Could you check a few things on this model? Use its own coordinates, in mm. A direction names the side the tool comes from. Coordinates: 2 decimals unless noted, no trailing zeros. Loops run counter-clockwise (first coordinate to the right, second up) from the corner with the lowest first, then second, coordinate; pieces in that order, holes last. Notation, with made-up numbers: (25, 67.25) - (31, 67.25) arc R5 ccw to (31, 75.25) - close; hole circle Ø6 at (68.25, 49.5). An arc over 180 degrees is marked (long way). Put each result on its own line as item: value. Start each with the question number.
```python
from build123d import *

# Parameters (mm, degrees)
SKETCH1_R           = 57
SKETCH1_R_2         = 2
SKETCH1_R_3         = 5.25
SKETCH1_R_4         = 10.75
BOSS_EXTRUDE1_DEPTH = 20
SKETCH2_R           = 57
SKETCH2_R_2         = 54
BOSS_EXTRUDE2_DEPTH = 130
SKETCH3_R           = 8
CUT_EXTRUDE1_DEPTH  = 19.5
SKETCH5_R           = 12
CUT_EXTRUDE3_DEPTH  = 6.05


with BuildPart() as part:
    # Sketch1 → Boss-Extrude1 (new body)
    with BuildSketch(Plane.XY):
        with Locations((0, 25)):
            Circle(SKETCH1_R)
        with Locations((12, 0)):
            Circle(SKETCH1_R_2, mode=Mode.SUBTRACT)
        with Locations((0, -12)):
            Circle(SKETCH1_R_2, mode=Mode.SUBTRACT)
        with Locations((-12, 0)):
            Circle(SKETCH1_R_2, mode=Mode.SUBTRACT)
        Circle(SKETCH1_R_3, mode=Mode.SUBTRACT)
        with Locations((0, 12)):
            Circle(SKETCH1_R_2, mode=Mode.SUBTRACT)
        with Locations((0, 50)):
            Circle(SKETCH1_R_4, mode=Mode.SUBTRACT)
    extrude(amount=-BOSS_EXTRUDE1_DEPTH)

    # Sketch2 → Boss-Extrude2 (add)
    with BuildSketch(Plane.XY):
        with Locations((0, 25)):
            Circle(SKETCH2_R)
        with Locations((0, 25)):
            Circle(SKETCH2_R_2, mode=Mode.SUBTRACT)
    extrude(amount=-BOSS_EXTRUDE2_DEPTH)

    # Sketch3 → Cut-Extrude1 (cut)
    with BuildSketch(Plane.XY):
        with Locations((40, 25)):
            Circle(SKETCH3_R)
    cut_extrude1 = extrude(amount=-CUT_EXTRUDE1_DEPTH, mode=Mode.SUBTRACT)

    # Sketch5 → Cut-Extrude3 (cut)
    with BuildSketch(Plane(origin=(0, 0, -20), x_dir=(-1, 0, 0), z_dir=(0, 0, -1))):
        with Locations((-40, 25)):
            Circle(SKETCH5_R)
    cut_extrude3 = extrude(amount=-CUT_EXTRUDE3_DEPTH, mode=Mode.SUBTRACT)

    # Mirror1: Cut-Extrude1, Cut-Extrude3 across plane
    add(cut_extrude1.mirror(Plane(origin=(0, 0, 0), x_dir=(0, 0, 1), z_dir=(1, 0, 0))), mode=Mode.SUBTRACT)
    add(cut_extrude3.mirror(Plane(origin=(0, 0, 0), x_dir=(0, 0, 1), z_dir=(1, 0, 0))), mode=Mode.SUBTRACT)


solid = part.part
```
(1) I want a section at A-A on x = 0. List the corners of the cut face in (y, z) for me.
(2) Which directions (+Z, -Z, +X, -X, +Y, -Y) give clear straight access to the entire face, cutting with the end or side of a thin tool? Please do faces 1 (the cylindrical face through (-49.523, 17.698, -17.017)), 2 (the cylindrical face through (0, 14, -10)).
(3) I need wall thicknesses on L1, parallel to Y at x = 0, z = -10.25; L2, parallel to X at y = -1, z = -14; L3, parallel to Y at x = -1, z = -10. Which ranges of each line are inside material? Lowest first, please. Write a range as [from, to].
(4) For pin 1 Ø8 at (y, z) = (59, -96) entering from -X; pin 2 Ø9.5 at (x, y) = (-40, 25) entering from +Z; pin 3 Ø4 at (x, z) = (-24, -33) entering from +Y; pin 4 Ø6.5 at (x, y) = (-12, 0) entering from -Z, each with a flat end and sliding along its axis, tell me the tip position at first contact or that it passes through.
(5) I want a section at C-C on x = -41.5. List the corners of the cut face in (y, z) for me, and give its area (3 significant figures).
(6) I want a section at B-B on y = 41. List the corners of the cut face in (x, z) for me.
(7) I want a section at D-D on z = -92. List the corners of the cut face in (x, y) for me.
(8) If we mould it in two halves opening along X, with no side actions, what happens to faces 3 (the flat face through (32, 23, -13.95)), 4 (the cylindrical face through (-12.356, -30.645, -64.09)), 5 (the flat face through (50, 4, -130))? For each: pulls with the +X half, pulls with the -X half, needs draft (parallel to the pull), parting line crosses it, or undercut.
Answer sheet:
1. outline: (-32, -130) - (-29, -130) - (-29, -20) - (-14, -20) - (-14, 0) - (-32, 0) - close; (-10, -20) - (-5.25, -20) - (-5.25, 0) - (-10, 0) - close; (5.25, -20) - (10, -20) - (10, 0) - (5.25, 0) - close; (14, -20) - (39.25, -20) - (39.25, 0) - (14, 0) - close; (60.75, -20) - (79, -20) - (79, -130) - (82, -130) - (82, 0) - (60.75, 0) - close
2. face 1: -Z
2. face 2: +Z, -Z
3. L1: y = [-32, -14], [-10, -5.25], [5.25, 10], [14, 39.25], [60.75, 82]
3. L2: x = [-50.72, -13.73], [-10.27, -5.15], [5.15, 10.27], [13.73, 50.72]
3. L3: y = [-31.99, -13.73], [-10.27, -5.15], [5.15, 10.27], [13.73, 39.3], [60.7, 81.99]
4. pin 1: stops at x = -48.47
4. pin 2: passes through
4. pin 3: stops at y = 77.58
4. pin 4: stops at z = -20
5. outline: (-14.07, -130) - (-9.55, -130) - (-9.55, -20) - (13.09, -20) - (13.09, -13.95) - (17.14, -13.95) - (17.14, 0) - (-14.07, 0) - close; (32.86, -13.95) - (36.91, -13.95) - (36.91, -20) - (59.55, -20) - (59.55, -130) - (64.07, -130) - (64.07, 0) - (32.86, 0) - close
5. area: 2,190 mm^2
6. outline: (-54.71, -130) - (-51.58, -130) - (-51.58, -20) - (-5.88, -20) - (-5.88, 0) - (-54.71, 0) - close; (5.88, -20) - (51.58, -20) - (51.58, -130) - (54.71, -130) - (54.71, 0) - (5.88, 0) - close
7. outline: circle Ø114 at (0, 25); hole circle Ø108 at (0, 25)
8. face 3: undercut
8. face 4: parting line crosses it
8. face 5: needs draft
